from build123d import *

# Parameters (mm, degrees)
SKETCH_1_R      = 2.6
EXTRUDE_2_DEPTH = 300


with BuildPart() as part:
    # 草图1 → 凸台-拉伸2 (new body)
    with BuildSketch(Plane(origin=(0, 170, 0), x_dir=(1, 0, 0), z_dir=(0, 1, 0))):
        with BuildLine():
            Line((-3.1, 8.85), (-3.1, 9.5))
            ThreePointArc((-3.1, 9.5), (-3.246446609, 9.853553391), (-3.6, 10))
            Line((-3.6, 10), (-9, 10))
            ThreePointArc((-9, 10), (-9.707106781, 9.707106781), (-10, 9))
            Line((-10, 9), (-10, 3.6))
            ThreePointArc((-10, 3.6), (-9.853553391, 3.246446609), (-9.5, 3.1))
            Line((-9.5, 3.1), (-8.85, 3.1))
            ThreePointArc((-8.85, 3.1), (-8.496446609, 3.246446609), (-8.35, 3.6))
            Line((-8.35, 3.6), (-8.35, 5))
            ThreePointArc((-8.35, 5), (-8.203553391, 5.353553391), (-7.85, 5.5))
            Line((-7.85, 5.5), (-6.626345597, 5.5))
            ThreePointArc((-6.626345597, 5.5), (-6.435003881, 5.461939766), (-6.272792206, 5.353553391))
            Line((-6.272792206, 5.353553391), (-4.046446609, 3.127207794))
            ThreePointArc((-4.046446609, 3.127207794), (-3.938060234, 2.964996119), (-3.9, 2.773654403))
            Line((-3.9, 2.773654403), (-3.9, -2.773654403))
            ThreePointArc((-3.9, -2.773654403), (-3.938060234, -2.964996119), (-4.046446609, -3.127207794))
            Line((-4.046446609, -3.127207794), (-6.272792206, -5.353553391))
            ThreePointArc((-6.272792206, -5.353553391), (-6.435003881, -5.461939766), (-6.626345597, -5.5))
            Line((-6.626345597, -5.5), (-7.85, -5.5))
            ThreePointArc((-7.85, -5.5), (-8.203553391, -5.353553391), (-8.35, -5))
            Line((-8.35, -5), (-8.35, -3.6))
            ThreePointArc((-8.35, -3.6), (-8.496446609, -3.246446609), (-8.85, -3.1))
            Line((-8.85, -3.1), (-9.5, -3.1))
            ThreePointArc((-9.5, -3.1), (-9.853553391, -3.246446609), (-10, -3.6))
            Line((-10, -3.6), (-10, -9))
            ThreePointArc((-10, -9), (-9.707106781, -9.707106781), (-9, -10))
            Line((-9, -10), (-3.6, -10))
            ThreePointArc((-3.6, -10), (-3.246446609, -9.853553391), (-3.1, -9.5))
            Line((-3.1, -9.5), (-3.1, -8.85))
            ThreePointArc((-3.1, -8.85), (-3.246446609, -8.496446609), (-3.6, -8.35))
            Line((-3.6, -8.35), (-5, -8.35))
            ThreePointArc((-5, -8.35), (-5.353553391, -8.203553391), (-5.5, -7.85))
            Line((-5.5, -7.85), (-5.5, -6.626345597))
            ThreePointArc((-5.5, -6.626345597), (-5.461939766, -6.435003881), (-5.353553391, -6.272792206))
            Line((-5.353553391, -6.272792206), (-3.127207794, -4.046446609))
            ThreePointArc((-3.127207794, -4.046446609), (-2.964996119, -3.938060234), (-2.773654403, -3.9))
            Line((-2.773654403, -3.9), (2.773654403, -3.9))
            ThreePointArc((2.773654403, -3.9), (2.964996119, -3.938060234), (3.127207794, -4.046446609))
            Line((3.127207794, -4.046446609), (5.353553391, -6.272792206))
            ThreePointArc((5.353553391, -6.272792206), (5.461939766, -6.435003881), (5.5, -6.626345597))
            Line((5.5, -6.626345597), (5.5, -7.85))
            ThreePointArc((5.5, -7.85), (5.353553391, -8.203553391), (5, -8.35))
            Line((5, -8.35), (3.6, -8.35))
            ThreePointArc((3.6, -8.35), (3.246446609, -8.496446609), (3.1, -8.85))
            Line((3.1, -8.85), (3.1, -9.5))
            ThreePointArc((3.1, -9.5), (3.246446609, -9.853553391), (3.6, -10))
            Line((3.6, -10), (9, -10))
            ThreePointArc((9, -10), (9.707106781, -9.707106781), (10, -9))
            Line((10, -9), (10, -3.6))
            ThreePointArc((10, -3.6), (9.853553391, -3.246446609), (9.5, -3.1))
            Line((9.5, -3.1), (8.85, -3.1))
            ThreePointArc((8.85, -3.1), (8.496446609, -3.246446609), (8.35, -3.6))
            Line((8.35, -3.6), (8.35, -5))
            ThreePointArc((8.35, -5), (8.203553391, -5.353553391), (7.85, -5.5))
            Line((7.85, -5.5), (6.626345597, -5.5))
            ThreePointArc((6.626345597, -5.5), (6.435003881, -5.461939766), (6.272792206, -5.353553391))
            Line((6.272792206, -5.353553391), (4.046446609, -3.127207794))
            ThreePointArc((4.046446609, -3.127207794), (3.938060234, -2.964996119), (3.9, -2.773654403))
            Line((3.9, -2.773654403), (3.9, 2.773654403))
            ThreePointArc((3.9, 2.773654403), (3.938060234, 2.964996119), (4.046446609, 3.127207794))
            Line((4.046446609, 3.127207794), (6.272792206, 5.353553391))
            ThreePointArc((6.272792206, 5.353553391), (6.435003881, 5.461939766), (6.626345597, 5.5))
            Line((6.626345597, 5.5), (7.85, 5.5))
            ThreePointArc((7.85, 5.5), (8.203553391, 5.353553391), (8.35, 5))
            Line((8.35, 5), (8.35, 3.6))
            ThreePointArc((8.35, 3.6), (8.496446609, 3.246446609), (8.85, 3.1))
            Line((8.85, 3.1), (9.5, 3.1))
            ThreePointArc((9.5, 3.1), (9.853553391, 3.246446609), (10, 3.6))
            Line((10, 3.6), (10, 9))
            ThreePointArc((10, 9), (9.707106781, 9.707106781), (9, 10))
            Line((9, 10), (3.6, 10))
            ThreePointArc((3.6, 10), (3.246446609, 9.853553391), (3.1, 9.5))
            Line((3.1, 9.5), (3.1, 8.85))
            ThreePointArc((3.1, 8.85), (3.246446609, 8.496446609), (3.6, 8.35))
            Line((3.6, 8.35), (5, 8.35))
            ThreePointArc((5, 8.35), (5.353553391, 8.203553391), (5.5, 7.85))
            Line((5.5, 7.85), (5.5, 6.626345597))
            ThreePointArc((5.5, 6.626345597), (5.461939766, 6.435003881), (5.353553391, 6.272792206))
            Line((5.353553391, 6.272792206), (3.127207794, 4.046446609))
            ThreePointArc((3.127207794, 4.046446609), (2.964996119, 3.938060234), (2.773654403, 3.9))
            Line((2.773654403, 3.9), (-2.773654403, 3.9))
            ThreePointArc((-2.773654403, 3.9), (-2.964996119, 3.938060234), (-3.127207794, 4.046446609))
            Line((-3.127207794, 4.046446609), (-5.5, 6.419238816))
            Line((-5.5, 6.419238816), (-5.5, 7.85))
            ThreePointArc((-5.5, 7.85), (-5.353553391, 8.203553391), (-5, 8.35))
            Line((-5, 8.35), (-3.6, 8.35))
            ThreePointArc((-3.6, 8.35), (-3.246446609, 8.496446609), (-3.1, 8.85))
        make_face()
        with Locations(Location((0, 0, 0), (0, 0, 90))):
            Circle(SKETCH_1_R, mode=Mode.SUBTRACT)
    extrude(amount=EXTRUDE_2_DEPTH)


solid = part.part
The listing builds one solid part. Answer for the finished solid, in the listing's coordinates (mm). A direction names the side the tool comes from. Coordinates: 2 decimals unless noted, no trailing zeros. Loops run counter-clockwise (first coordinate to the right, second up) from the corner with the lowest first, then second, coordinate; pieces in that order, holes last. Notation, with made-up numbers: M 13.5,40 L 30.5,40 A20 cw 30.5,71 Z; hole C 70,71 d3. An arc over 180 degrees is marked long. Answer in a Markdown table with one row per item.
1) Which of the six approach directions +Z, -Z, +X, -X, +Y, -Y give full straight-line access (tool end or side, diameter ignored) to faces 1 (the flat face through (0, 318, -3.9)), 2 (the flat face through (-10, 318, -6)), 3 (the flat face through (0, 318, 3.9)), 4 (the flat face through (3.9, 318, 0))?
Answers below:
| item | result |
|---|---|
| face 1 | -Z, +Y, -Y |
| face 2 | +Z, -Z, -X, +Y, -Y |
| face 3 | +Z, +Y, -Y |
| face 4 | +X, +Y, -Y |
2) Determine the mould class of faces 5 (the flat face through (-3.9, 318, 0)), 6 (the cylindrical face through (-0.78, 317.9, -2.48)), 7 (the flat face through (6, 318, 10)) for opening direction X: released by +X, released by -X, zero draft, split by the parting line, or undercut.
Answers below:
| item | result |
|---|---|
| face 5 | released by -X |
| face 6 | undercut |
| face 7 | zero draft |
3) Given pin 1 (0.7 mm diameter, centred on x = -9.5, y = 262.5, fed in from +Z); pin 2 (1.7 mm diameter, centred on y = 281, z = 0, fed in from +X); pin 3 (2 mm diameter, centred on x = -7, z = -2, fed in from -Y); pin 4 (6 mm diameter, centred on y = 250, z = -0.5, fed in from -X), each flat-ended and moving along its own axis, determine where each tip first touches the part or whether it passes through.
Answers below:
| item | result |
|---|---|
| pin 1 | z = 9.99 |
| pin 2 | x = 3.9 |
| pin 3 | through |
| pin 4 | x = -9.99 |
4) Find section B-B (x = 0). Determine the outline of the cut face in (y, z).
Answers below:
| item | result |
|---|---|
| outline | M 170,-3.9 L 470,-3.9 L 470,-2.6 L 170,-2.6 Z; M 170,2.6 L 470,2.6 L 470,3.9 L 170,3.9 Z |
5) Find the intervals of material crossed by probe 1 along X at (y, z) = (322, -8); probe 2 along Z at (x, y) = (4.25, 329.5); probe 3 along Z at (x, y) = (3.75, 203), in increasing order.
Answers below:
| item | result |
|---|---|
| probe 1 | -10 to -5.48, 5.48 to 10 |
| probe 2 | -10 to -8.35, -5.17 to -3.33, 3.33 to 5.17, 8.35 to 10 |
| probe 3 | -10 to -8.35, -4.67 to 4.67, 8.35 to 10 |
6) Find section A-A (z = 0). Determine the outline of the cut face in (x, y), then the cut area to 3 significant figures.
Answers below:
| item | result |
|---|---|
| outline | M -3.9,170 L -2.6,170 L -2.6,470 L -3.9,470 Z; M 2.6,170 L 3.9,170 L 3.9,470 L 2.6,470 Z |
| area | 780 mm^2 |
